Work out the finished part from the listing and answer in its coordinate system (mm). Give positions to 0.01 mm unless a question says otherwise; leave off trailing zeros. Write each loop counter-clockwise with the first axis right and the second up, starting at its lowest first coordinate (ties: lowest second). Pieces come first, ordered by that corner, then holes.
1) Given pin 1 Ø1.5 at (y, z) = (141, 1) entering from +X; pin 2 Ø0.9 at (y, z) = (189, 2) entering from -X; pin 3 Ø1.5 at (x, z) = (12, 2) entering from +Y, each flat-ended and moving along its own axis, determine where each tip first touches the part or whether it passes through.
2) Find section A-A (y = 146). Determine the outline of the cut face in (x, z).
3) Straight lines are drawn through the part: probe 1 along X at (y, z) = (224.5, 1.6); probe 2 along Y at (x, z) = (10.5, 0.8). For each, find the intervals that lie inside material, in ascending order.
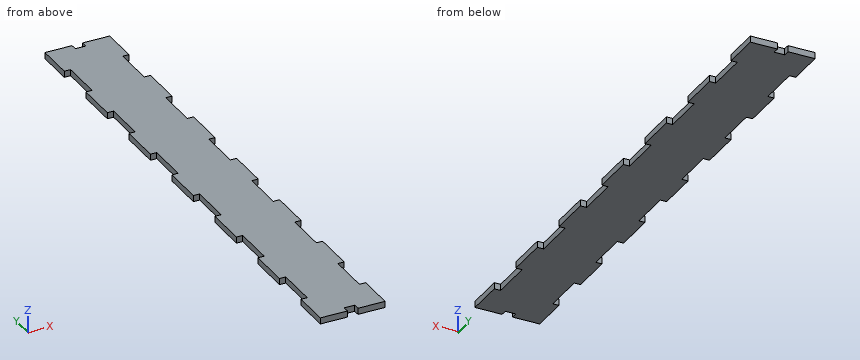
```python
from build123d import *

# Parameters (mm, degrees)
BOSS_EXTRUDE3_DEPTH = 3


with BuildPart() as part:
    # Sketch2 → Boss-Extrude3 (new body)
    with BuildSketch(Plane.XY):
        Polygon((10, 250), (15, 250), (15, 253), (25, 253), (28, 253), (28, 235), (25, 235), (25, 215), (28, 215), (28, 195), (25, 195), (25, 175), (28, 175), (28, 155), (25, 155), (25, 135), (28, 135), (28, 115), (25, 115), (25, 95), (28, 95), (28, 75), (25, 75), (25, 55), (28, 55), (28, 35), (25, 35), (25, 15), (28, 15), (28, -3), (25, -3), (15, -3), (15, 0), (10, 0), (10, -3), (0, -3), (-3, -3), (-3, 15), (0, 15), (0, 35), (-3, 35), (-3, 55), (0, 55), (0, 75), (-3, 75), (-3, 95), (0, 95), (0, 115), (-3, 115), (-3, 135), (0, 135), (0, 155), (-3, 155), (-3, 175), (0, 175), (0, 195), (-3, 195), (-3, 215), (0, 215), (0, 235), (-3, 235), (-3, 253), (0, 253), (10, 253), align=None)
    extrude(amount=BOSS_EXTRUDE3_DEPTH)


solid = part.part
```
Results:
1. pin 1: stops at x = 25
1. pin 2: stops at x = 0
1. pin 3: stops at y = 250
2. outline: (0, 0) - (25, 0) - (25, 3) - (0, 3) - close
3. probe 1: x = 0 to 25
3. probe 2: y = 0 to 250
